from build123d import *

# Parameters (mm, degrees)
F1_DEPTH = 40
F3_DEPTH = 30
F4_R     = 5


with BuildPart() as f1:
    # F0 (on Top) → F1 (new body)
    with BuildSketch(Plane.XY):
        with BuildLine():
            ThreePointArc((0, 5), (1.4644660941, 1.4644660941), (5, 0))
            Line((5, 0), (155, 0))
            ThreePointArc((155, 0), (158.5355339059, 1.4644660941), (160, 5))
            Line((160, 5), (160, 95))
            ThreePointArc((160, 95), (158.5355339059, 98.5355339059), (155, 100))
            Line((155, 100), (5, 100))
            ThreePointArc((5, 100), (1.4644660941, 98.5355339059), (0, 95))
            Line((0, 95), (0, 5))
        make_face()
    extrude(amount=F1_DEPTH)

    # F2 (on face) → F3 (cut)
    with BuildSketch(Plane.XY.offset(40)):
        with BuildLine():
            Line((140, 85), (20, 85))
            ThreePointArc((20, 85), (16.4644660941, 83.5355339059), (15, 80))
            Line((15, 80), (15, 20))
            ThreePointArc((15, 20), (16.4644660941, 16.4644660941), (20, 15))
            Line((20, 15), (140, 15))
            ThreePointArc((140, 15), (143.5355339059, 16.4644660941), (145, 20))
            Line((145, 20), (145, 80))
            ThreePointArc((145, 80), (143.5355339059, 83.5355339059), (140, 85))
        make_face()
    extrude(amount=-F3_DEPTH, mode=Mode.SUBTRACT)

    # F4
    f4_edges = [f1.edges().sort_by_distance(p)[0] for p in [
        (80, 85, 10),
        (0, 50, 40),
        (1.464466, 98.535534, 40),
        (1.464466, 1.464466, 40),
        (80, 100, 40),
        (80, 0, 40),
        (158.535534, 98.535534, 40),
        (158.535534, 1.464466, 40),
        (160, 50, 40),
        (80, 85, 40),
        (16.464466, 83.535534, 40),
        (15, 50, 40),
        (16.464466, 16.464466, 40),
        (80, 15, 40),
        (143.535534, 16.464466, 40),
        (145, 50, 40),
        (143.535534, 83.535534, 40),
    ]]
    fillet(f4_edges, radius=F4_R)


solid = f1.part
Could you check a few things on this model? Use its own coordinates, in mm. A direction names the side the tool comes from. Give positions to 0.01 mm unless a question says otherwise; leave off trailing zeros. Loops run counter-clockwise (first coordinate to the right, second up) from the corner with the lowest first, then second, coordinate; pieces in that order, holes last. Notation, with made-up numbers: M 15.5,35 L 48.5,35 A22 ccw 48.5,69 Z; hole C 47,0.25 d4. An arc over 180 degrees is marked long. Answer as a JSON object with one key per item and string values.
Q1. For P1, Ø1, axis at x = 48.5, y = 81.5, coming from the +Z side, with a flat end and sliding along its axis, tell me the tip position at first contact or that it passes through.
Values found:
{"P1": "stops at z = 10.42"}
Q2. Suppose I cut it at C-C, the plane y = 75. List the corners of the cut face in (x, z) for me, plus the area to 3 significant figures.
Values found:
{"outline": "M 0,0 L 160,0 L 160,35 A5 ccw 155,40 L 150,40 A5 ccw 145,35 L 145,15 A5 cw 140,10 L 20,10 A5 cw 15,15 L 15,35 A5 ccw 10,40 L 5,40 A5 ccw 0,35 Z", "area": "2,490 mm²"}
Q3. If I drill on probe 1 along X at (y, z) = (55.5, 21.5); probe 2 along Y at (x, z) = (42.5, 17.5); probe 3 along Z at (x, y) = (38, 57.5), over which ranges is the centre line in solid material (lowest first)? Write a range as [from, to].
Values found:
{"probe 1": "x = [0, 15], [145, 160]", "probe 2": "y = [0, 15], [85, 100]", "probe 3": "z = [0, 10]"}
Q4. For faces 4 (the flat face through (79.6, 90.2, 40)), 5 (the flat face through (81, 85, 25)), which set-ups out of +Z, -Z, +X, -X, +Y, -Y let a thin tool reach every point of the face, with its end or its side?
Values found:
{"face 4": "+Z, +X, -X, +Y, -Y", "face 5": "+Z"}
Q5. Suppose I cut it at A-A, the plane x = 32.5. List the corners of the cut face in (y, z) for me, plus the area to 3 significant figures.
Values found:
{"outline": "M 0,0 L 100,0 L 100,35 A5 ccw 95,40 L 90,40 A5 ccw 85,35 L 85,15 A5 cw 80,10 L 20,10 A5 cw 15,15 L 15,35 A5 ccw 10,40 L 5,40 A5 ccw 0,35 Z", "area": "1,890 mm²"}
Q6. Suppose I cut it at B-B, the plane z = 18. List the corners of the cut face in (x, y) for me, plus the area to 3 significant figures.
Values found:
{"outline": "M 0,5 A5 ccw 5,0 L 155,0 A5 ccw 160,5 L 160,95 A5 ccw 155,100 L 5,100 A5 ccw 0,95 Z; hole M 15,20 A5 ccw 20,15 L 140,15 A5 ccw 145,20 L 145,80 A5 ccw 140,85 L 20,85 A5 ccw 15,80 Z", "area": "6,900 mm²"}
Q7. If we mould it in two halves opening along Y, with no side actions, what happens to faces 1 (the cylindrical face through (147, 50, 39)), 2 (the cylindrical face through (158, 1, 17)), 3 (the flat face through (81, 100, 17))? For each: pulls with the +Y half, pulls with the -Y half, needs draft (parallel to the pull), parting line crosses it, or undercut.
Values found:
{"face 1": "undercut", "face 2": "pulls with the -Y half", "face 3": "pulls with the +Y half"}
Q8. Suppose I cut it at D-D, the plane z = 37.5. List the corners of the cut face in (x, y) for me, plus the area to 3 significant figures.
Values found:
{"outline": "M 0.67,5 A4.33 ccw 5,0.67 L 155,0.67 A4.33 ccw 159.33,5 L 159.33,95 A4.33 ccw 155,99.33 L 5,99.33 A4.33 ccw 0.67,95 Z; hole M 14.33,20 A5.67 ccw 20,14.33 L 140,14.33 A5.67 ccw 145.67,20 L 145.67,80 A5.67 ccw 140,85.67 L 20,85.67 A5.67 ccw 14.33,80 Z", "area": "6,300 mm²"}
